```python
from build123d import *

# Parameters (mm, degrees)
SHELL2_START       = 1.524
SHELL2_OUTLINE_R   = 176.276
SHELL2_DEPTH       = 289.052
SHELL2_START_2     = 290.576
SHELL2_2_OUTLINE_R = 36.576
SHELL2_2_DEPTH     = 52.324
CUT_EXTRUDE1_REACH = 427.213
SKETCH2_R          = 2.999994
CIRPATTERN1_COUNT  = 4


# Read off the part's stored shape, not the designer's step: Shell2
with BuildPart() as part:
    # Sketch1 → Revolve1 (revolve)
    with BuildSketch(Plane.XY, mode=Mode.PRIVATE) as revolve1_sk:
        Polygon((0, 0), (177.8, 0), (177.8, 292.1), (38.1, 292.1), (38.1, 341.376), (63.5, 341.376), (63.5, 342.9), (0, 342.9), align=None)
    revolve(revolve1_sk.sketch.rotate(Axis((0, 342.9, 0), (0, -1, 0)), 180), axis=Axis((0, 342.9, 0), (0, -1, 0)))

    # Shell2 outline → Shell2 (cut)
    with BuildSketch(Plane(origin=(0, 0, 0), x_dir=(1, 0, 0), z_dir=(0, 1, 0)).offset(SHELL2_START)):
        Circle(SHELL2_OUTLINE_R)
    extrude(amount=SHELL2_DEPTH, mode=Mode.SUBTRACT)

    # Shell2 2 outline → Shell2 2 (cut)
    with BuildSketch(Plane(origin=(0, 0, 0), x_dir=(1, 0, 0), z_dir=(0, 1, 0)).offset(SHELL2_START_2)):
        Circle(SHELL2_2_OUTLINE_R)
    extrude(amount=SHELL2_2_DEPTH, mode=Mode.SUBTRACT)

    # Sketch2 → Cut-Extrude1 (cut, up to next)
    with BuildSketch(Plane(origin=(0, 342.9, 0), x_dir=(1, 0, 0), z_dir=(0, 1, 0)), mode=Mode.PRIVATE) as cut_extrude1_sk1:
        with Locations(Location((50.8, 0, 0), (0, 0, 180))):
            Circle(SKETCH2_R)
    cut_extrude1_tool1 = extrude(cut_extrude1_sk1.sketch, amount=-CUT_EXTRUDE1_REACH, mode=Mode.PRIVATE) & part.part
    cut_extrude1 = cut_extrude1_tool1.solids().sort_by_distance((50.8, 342.9, 0))[0]
    add(cut_extrude1, mode=Mode.SUBTRACT)

    # CirPattern1: Cut-Extrude1 ×4 about axis
    cirpattern1_axis = Axis((0, 0, 0), (0, 1, 0))
    for i in range(1, CIRPATTERN1_COUNT):
        add(cut_extrude1.rotate(cirpattern1_axis, i * 360 / CIRPATTERN1_COUNT), mode=Mode.SUBTRACT)


solid = part.part
```
Work out the finished part from the listing and answer in its coordinate system (mm). A direction names the side the tool comes from. Coordinates: 2 decimals unless noted, no trailing zeros. Loops run counter-clockwise (first coordinate to the right, second up) from the corner with the lowest first, then second, coordinate; pieces in that order, holes last. Notation, with made-up numbers: M 28,56.5 L 69,56.5 A22 cw 69,92.5 Z; hole C -31,-27 d6. An arc over 180 degrees is marked long. Use CSV: the item, a comma, the result in double quotes. Start each with the question number.
(1) For faces 4 (the face through (13.77, 342.15, 61.99)), 5 (the face through (-2, 1.524, -2)), 6 (the face through (-2, 0, -2)), determine the directions among +Z, -Z, +X, -X, +Y, -Y from which every point of the face is accessible in a straight line to the end or side of a thin tool.
(2) Find section A-A, the plane x = 87.5. Give the vertices of the cut face in (y, z), then the cut area to 3 significant figures.
(3) Consider line 1 (Y direction, x = -16.5, z = 54); line 2 (Y direction, x = 44, z = 58); line 3 (Z direction, x = 0, y = 116.5). Determine where each line is inside the solid, lowest interval first.
(4) Given pin 1 Ø12 at (x, z) = (-104.5, 71) entering from -Y; pin 2 Ø4 at (x, y) = (105, 89) entering from -Z; pin 3 Ø5 at (x, z) = (50.8, 0) entering from +Y; pin 4 Ø10 at (x, y) = (44.5, 60.5) entering from +Z, each flat-ended and moving along its own axis, determine where each tip first touches the part or whether it passes through.
(5) Find section B-B, the plane z = -148. Give the vertices of the cut face in (x, y), then the cut area to 3 significant figures.
(6) Find section C-C, the plane y = 32. Give the vertices of the cut face in (x, z), then the cut area to 3 significant figures.
(7) For a pull along Y with two mould halves and no side action, classify faces 1 (the face through (131.046, 148.095, -120.166)), 2 (the face through (-27, 342.9, 27)), 3 (the face through (-22.948, 144.027, -174.776)) as +Y half, -Y half, draft (parallel to the pull), parting line (faces both ways), or undercut.
(8) Find section D-D, the plane x = 25. Give the vertices of the cut face in (y, z).
Recorded:
1,face 4,"+Y"
1,face 5,"none"
1,face 6,"+Z, -Z, +X, -X, -Y"
2,outline,"M 0,-154.78 L 292.1,-154.78 L 292.1,154.78 L 0,154.78 Z; hole M 1.52,-153.03 L 290.58,-153.03 L 290.58,153.03 L 1.52,153.03 Z"
2,area,"1,960 mm^2"
3,line 1,"y = 0 to 1.52, 290.58 to 292.1, 341.38 to 342.9"
3,line 2,"y = 0 to 1.52, 290.58 to 292.1"
3,line 3,"z = -177.8 to -176.28, 176.28 to 177.8"
4,pin 1,"stops at y = 0"
4,pin 2,"stops at z = -144.93"
4,pin 3,"stops at y = 292.1"
4,pin 4,"stops at z = 173.36"
5,outline,"M -98.53,0 L 98.53,0 L 98.53,292.1 L -98.53,292.1 Z; hole M -95.76,1.52 L 95.76,1.52 L 95.76,290.58 L -95.76,290.58 Z"
5,area,"2,210 mm^2"
6,outline,"C 0,0 d355.6; hole C 0,0 d352.55"
6,area,"1,700 mm^2"
7,face 1,"draft"
7,face 2,"+Y half"
7,face 3,"undercut"
8,outline,"M 0,-176.03 L 292.1,-176.03 L 292.1,-28.75 L 341.38,-28.75 L 341.38,-58.37 L 342.9,-58.37 L 342.9,-26.7 L 290.58,-26.7 L 290.58,-174.49 L 1.52,-174.49 L 1.52,174.49 L 290.58,174.49 L 290.58,26.7 L 342.9,26.7 L 342.9,58.37 L 341.38,58.37 L 341.38,28.75 L 292.1,28.75 L 292.1,176.03 L 0,176.03 Z"
